Verification items for this drawing (mm, ordinates from the low corner). Give positions to 0.01 mm unless a question says otherwise; leave off trailing zeros. Loops run counter-clockwise (first coordinate to the right, second up) from the corner with the lowest first, then second, coordinate; pieces in that order, holes last. Notation, with made-up numbers: (-32.5, -5.75) -> (-26.5, -5.75) arc R18 ccw to (-26.5, 10.25) -> close; hole circle Ø6 at (12, 28). An arc over 180 degrees is marked (long way). Write each question's results on one line, items separated by ' | '. Start each with the question number.
1) Sectioned sample at C-C on z = 101. Record the cut outline in (x, y).
2) Scan lines: line 1 (Z direction, x = 34, y = 2.75); line 2 (X direction, y = 0.55, z = 30); line 3 (Z direction, x = 36.5, y = 1.15). Record each from-to range of solid material in increasing order. Write a range as from..to.
3) Sectioned sample at D-D on x = 11.5. Record the cut outline in (y, z), then the cut area to 3 significant figures.
4) Sectioned sample at A-A on y = 2.4. Record the cut outline in (x, z), then the cut area to 3 significant figures.
5) Sectioned sample at B-B on x = 18. Record the cut outline in (y, z).
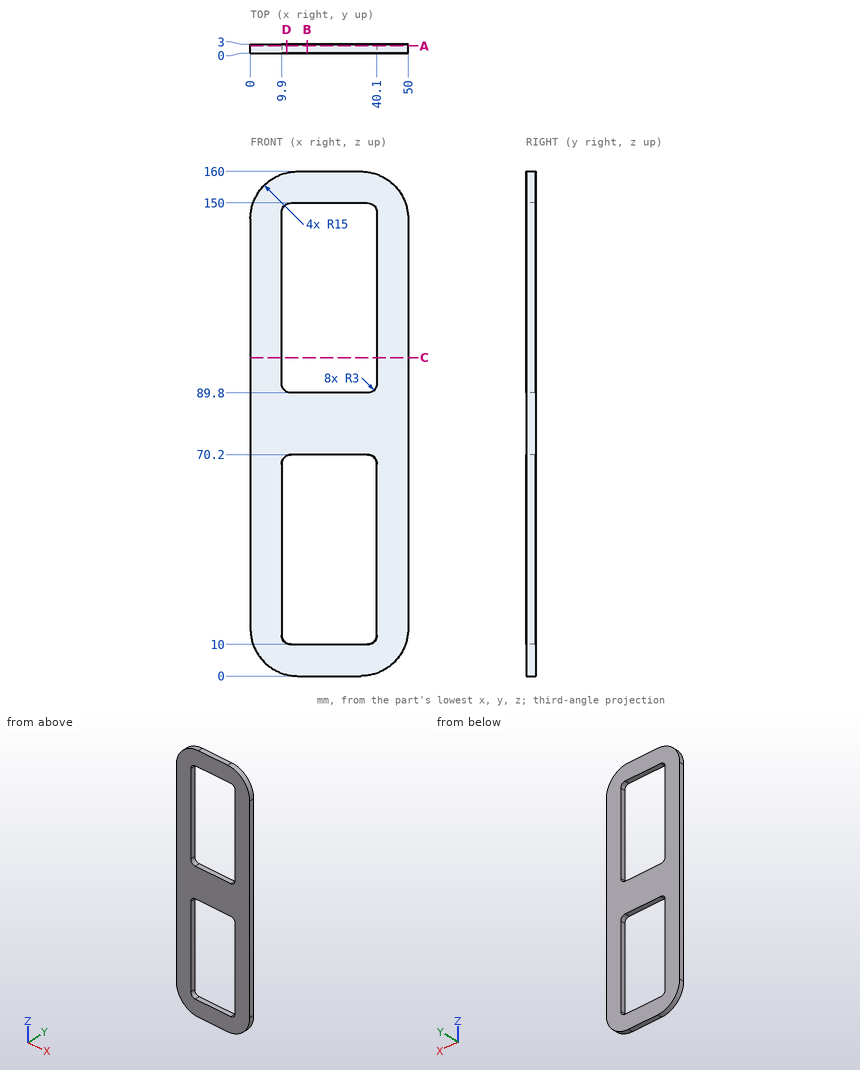
Result:
1) outline: (0, 0) -> (9.9, 0) -> (9.9, 3) -> (0, 3) -> close; (40.1, 0) -> (50, 0) -> (50, 3) -> (40.1, 3) -> close
2) line 1: 0..10, 70.2..89.8, 150..160 | line 2: 0..9.9, 40.1..50 | line 3: 0.08..10, 70.2..89.8, 150..159.92
3) outline: (0, 0.41) -> (3, 0.41) -> (3, 10.35) -> (0, 10.35) -> close; (0, 69.85) -> (3, 69.85) -> (3, 90.15) -> (0, 90.15) -> close; (0, 149.65) -> (3, 149.65) -> (3, 159.59) -> (0, 159.59) -> close | area: 120 mm^2
4) outline: (0, 15) arc R15 ccw to (15, 0) -> (35, 0) arc R15 ccw to (50, 15) -> (50, 145) arc R15 ccw to (35, 160) -> (15, 160) arc R15 ccw to (0, 145) -> close; hole (9.9, 13) arc R3 ccw to (12.9, 10) -> (37.1, 10) arc R3 ccw to (40.1, 13) -> (40.1, 67.2) arc R3 ccw to (37.1, 70.2) -> (12.9, 70.2) arc R3 ccw to (9.9, 67.2) -> close; hole (9.9, 92.8) arc R3 ccw to (12.9, 89.8) -> (37.1, 89.8) arc R3 ccw to (40.1, 92.8) -> (40.1, 147) arc R3 ccw to (37.1, 150) -> (12.9, 150) arc R3 ccw to (9.9, 147) -> close | area: 4,190 mm^2
5) outline: (0, 0) -> (3, 0) -> (3, 10) -> (0, 10) -> close; (0, 70.2) -> (3, 70.2) -> (3, 89.8) -> (0, 89.8) -> close; (0, 150) -> (3, 150) -> (3, 160) -> (0, 160) -> close
